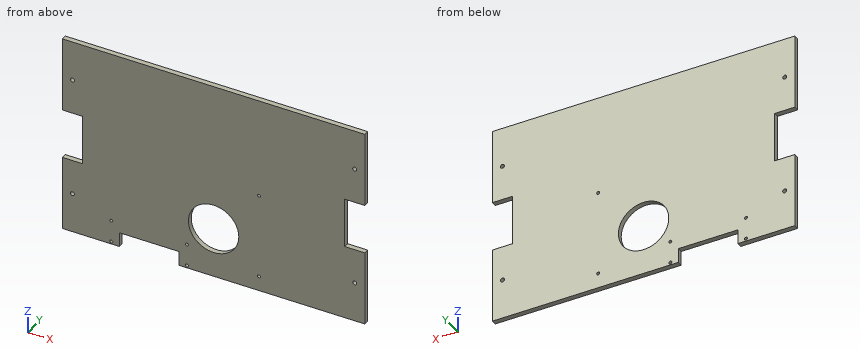
```python
from build123d import *

# Parameters (mm, degrees)
SKETCH1_W           = 300
SKETCH1_H           = 200
BOSS_EXTRUDE1_DEPTH = 5
SKETCH2_R           = 2
SKETCH2_R_2         = 25
CUT_EXTRUDE2_DEPTH  = 6
SKETCH4_R           = 1.5
CUT_EXTRUDE3_DEPTH  = 6
SKETCH6_W           = 59
SKETCH6_H           = 14.5
CUT_EXTRUDE4_DEPTH  = 5
SKETCH8_R           = 1.5
CUT_EXTRUDE6_DEPTH  = 6
SKETCH9_W           = 20
SKETCH9_H           = 50
CUT_EXTRUDE7_DEPTH  = 6


with BuildPart() as part:
    # Sketch1 → Boss-Extrude1 (new body)
    with BuildSketch(Plane(origin=(0, 0, 0), x_dir=(1, 0, 0), z_dir=(0, 1, 0))):
        Rectangle(SKETCH1_W, SKETCH1_H)
    extrude(amount=BOSS_EXTRUDE1_DEPTH)

    # Sketch2 → Cut-Extrude2 (cut, through all)
    with BuildSketch(Plane(origin=(0, 5, 0), x_dir=(1, 0, 0), z_dir=(0, 1, 0))):
        with Locations((-140, 0)):
            Circle(SKETCH2_R)
        with Locations((-140, 60)):
            Circle(SKETCH2_R)
        with Locations((-140, -60)):
            Circle(SKETCH2_R)
        with Locations((140, -60)):
            Circle(SKETCH2_R)
        with Locations((140, 60)):
            Circle(SKETCH2_R)
        with Locations((140, 0)):
            Circle(SKETCH2_R)
        with Locations((0, 50)):
            Circle(SKETCH2_R_2)
    extrude(amount=-CUT_EXTRUDE2_DEPTH, mode=Mode.SUBTRACT)

    # Sketch4 → Cut-Extrude3 (cut, through all)
    with BuildSketch(Plane(origin=(0, 5, 0), x_dir=(1, 0, 0), z_dir=(0, 1, 0))):
        with Locations((-101.5, 97.5)):
            Circle(SKETCH4_R)
        with Locations((-26.5, 97.5)):
            Circle(SKETCH4_R)
        with Locations((-26.5, 75.5)):
            Circle(SKETCH4_R)
        with Locations((-101.5, 75.5)):
            Circle(SKETCH4_R)
    extrude(amount=-CUT_EXTRUDE3_DEPTH, mode=Mode.SUBTRACT)

    # Sketch6 → Cut-Extrude4 (cut)
    with BuildSketch(Plane.XZ):
        with Locations((-64, -92.75)):
            Rectangle(SKETCH6_W, SKETCH6_H)
    extrude(amount=-CUT_EXTRUDE4_DEPTH, mode=Mode.SUBTRACT)

    # Sketch8 → Cut-Extrude6 (cut, through all)
    with BuildSketch(Plane(origin=(0, 5, 0), x_dir=(1, 0, 0), z_dir=(0, 1, 0))):
        with Locations((45, 85)):
            Circle(SKETCH8_R)
        with Locations((45, 0)):
            Circle(SKETCH8_R)
    extrude(amount=-CUT_EXTRUDE6_DEPTH, mode=Mode.SUBTRACT)

    # Sketch9 → Cut-Extrude7 (cut, through all)
    with BuildSketch(Plane(origin=(0, 5, 0), x_dir=(1, 0, 0), z_dir=(0, 1, 0))):
        with Locations((-140, 0)):
            Rectangle(SKETCH9_W, SKETCH9_H)
        with Locations((140, 0)):
            Rectangle(SKETCH9_W, SKETCH9_H)
    extrude(amount=-CUT_EXTRUDE7_DEPTH, mode=Mode.SUBTRACT)


solid = part.part
```
Read the model definition and answer for the solid it produces. Units are mm, in the model's axes. Coordinates: 2 decimals unless noted, no trailing zeros. Write each loop counter-clockwise with the first axis right and the second up, starting at its lowest first coordinate (ties: lowest second). Pieces come first, ordered by that corner, then holes. Notation, with made-up numbers: (8, 81.5) - (46, 81.5) arc R13 cw to (46, 102.5) - close; hole circle Ø6 at (30.5, -30.75). An arc over 180 degrees is marked (long way). Answer as a JSON object with one key per item and string values. Group by question number.
1. A cutting plane is placed at C-C (z = -37.5). Determine the outline of the cut face in (x, y), plus the area to 3 significant figures.
2. Each of these flat-tipped pins is pushed along its axis until it touches: P1, Ø6.5, axis at x = -140, z = -60, coming from the +Y side; P2, Ø3.5, axis at x = 140, z = -60, coming from the +Y side; P3, Ø2, axis at x = -64, y = 1.5, coming from the -Z side; P4, Ø1.5, axis at y = 1, z = -22.5, coming from the +X side. Where does it stop, or does it pass through?
3. Consider L1, parallel to Z at x = -140, y = 1.1; L2, parallel to Z at x = -26.5, y = 1.7; L3, parallel to Z at x = 45, y = 3.55. Determine where each line is inside the solid, lowest interval first. Write a range as [from, to].
4. A cutting plane is placed at A-A (x = 0). Determine the outline of the cut face in (y, z), plus the area to 3 significant figures.
5. A cutting plane is placed at D-D (x = -43). Determine the outline of the cut face in (y, z).
6. A cutting plane is placed at B-B (y = 0.9). Give the number of separate pieces and of enclosed holes in the cut face, plus the area to 3 significant figures.
Worked out:
{
 "1": {"outline": "(-150, 0) - (-21.65, 0) - (-21.65, 5) - (-150, 5) - close; (21.65, 0) - (150, 0) - (150, 5) - (21.65, 5) - close", "area": "1,280 mm²"},
 "2": {"P1": "stops at y = 5", "P2": "passes through", "P3": "stops at z = -85.5", "P4": "stops at x = 130"},
 "3": {"L1": "z = [-100, -62], [-58, -25], [25, 58], [62, 100]", "L2": "z = [-100, -99], [-96, -77], [-74, 100]", "L3": "z = [-100, -86.5], [-83.5, -1.5], [1.5, 100]"},
 "4": {"outline": "(0, -100) - (5, -100) - (5, -75) - (0, -75) - close; (0, -25) - (5, -25) - (5, 100) - (0, 100) - close", "area": "750 mm²"},
 "5": {"outline": "(0, -85.5) - (5, -85.5) - (5, 100) - (0, 100) - close"},
 "6": {"separate pieces": "1", "enclosed holes": "11", "area": "55,100 mm²"}
}
